The model under review builds one solid part; all positions refer to its coordinate system, in mm. Face numbers are marked on the shaded views. A direction names the side the tool comes from. Coordinates: 2 decimals unless noted, no trailing zeros. Loops run counter-clockwise (first coordinate to the right, second up) from the corner with the lowest first, then second, coordinate; pieces in that order, holes last. Notation, with made-up numbers: (23, 88) - (33, 88) arc R36 ccw to (33, 125) - close; hole circle Ø1 at (38, 28.25). An arc over 180 degrees is marked (long way). One line per item, written item: value. Start each with the question number.
1. We need section C-C, the plane x = -2. Give the boundary of the cut face in (y, z), then the cut area to 3 significant figures.
2. We need section A-A, the plane y = -11.25. Give the boundary of the cut face in (x, z).
3. We need section D-D, the plane z = -5. Give the boundary of the cut face in (x, y).
4. To check wall thickness, follow line 1 (Z direction, x = -2, y = -11.5); line 2 (Z direction, x = 1.5, y = -11); line 3 (Z direction, x = 1.5, y = -0.5). State the ranges of each line that lie inside material, in increasing order.
5. We need section B-B, the plane y = -6. Give the boundary of the cut face in (x, z), then the cut area to 3 significant figures.
6. For the marked faces 5, 6, 7 and 8, list the 3-axis set-ups (+Z, -Z, +X, -X, +Y, -Y) from which the entire face can be reached by the end or side of a thin tool; tool diameter is ignored.
7. Mouldability with a two-part tool opening along Z and no side actions: class the marked faces 1, 2, 3 and 4 as +Z half, -Z half, draft (parallel to the pull), parting line (faces both ways), or undercut.
8. Insertion check: P1, Ø5.5, axis at x = 1.5, z = 15, coming from the -Y side; P2, Ø2, axis at x = 0.78, z = 14.47, coming from the -Y side; P3, Ø1, axis at x = 6, y = -4, coming from the -Z side; P4, Ø2, axis at x = 0.5, z = 3.5, coming from the -Y side. Each pin has a flat end and moves straight along its axis. Give the tip position at first contact, or say it passes through.
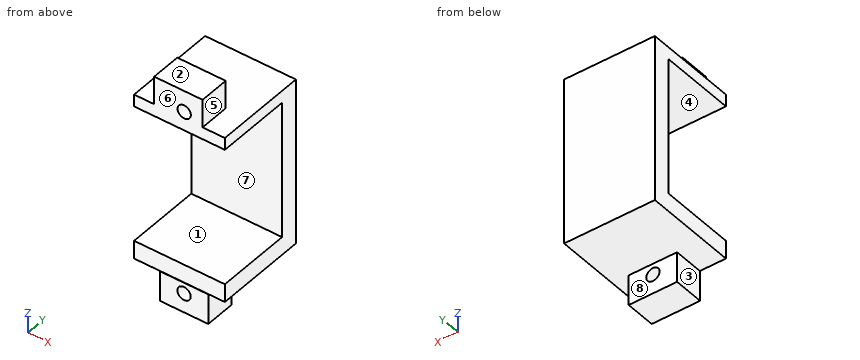
Autodesk Inventor part; units mm, degrees
ref_plane "YZ Plane" through (0, 0, 0) normal (1, 0, 0) x (0, 1, 0)
ref_plane "XZ Plane" through (0, 0, 0) normal (0, 1, 0) x (-1, 0, 0)
ref_plane "XY Plane" through (0, 0, 0) normal (0, 0, 1) x (1, 0, 0)
sketch "Sketch1" plane through (0, 0, 0) normal (0, 1, 0) x (-1, 0, 0)
  line L0 (7.5, 11.35) -> (-7.5, 11.35)
  line L1 (-7.5, 11.35) -> (-7.5, -11.35)
  line L2 (-7.5, -11.35) -> (7.5, -11.35)
  line L3 (7.5, -11.35) -> (7.5, 11.35)
  line L4 (7.5, 11.35) -> (-7.5, -11.35) construction
  line L5 (-7.5, 11.35) -> (7.5, -11.35) construction
  point P0 (0, 0)
  dimension "d0" = 15
  dimension "d1" = 22.7
extrude "Extrusion1" add sketch "Sketch1" along normal blind 3
sketch "Sketch2" plane through (0, 3, 0) normal (0, 1, 0) x (1, 0, 0)
  line L0 (-7.5, 11.35) -> (-7.5, -11.35)
  line L1 (-7.5, -11.35) -> (7.5, -11.35)
  line L2 (7.5, -11.35) -> (7.5, -13.35)
  line L3 (7.5, -13.35) -> (-7.5, -13.35)
  line L4 (-7.5, -13.35) -> (-7.5, -11.35)
  line L5 (-7.5, 11.35) -> (7.5, 11.35)
  line L6 (7.5, 11.35) -> (7.5, 14.35)
  line L7 (7.5, 14.35) -> (-7.5, 14.35)
  line L8 (-7.5, 14.35) -> (-7.5, 11.35)
  point P0 (0, 0)
  dimension "d4" = 15
  dimension "d5" = 2
  dimension "d6" = 3
extrude "Extrusion2" add sketch "Sketch2" against normal blind 15.4
sketch "Sketch3" plane through (-7.5, 3, 13.35) normal (0, 0, 1) x (1, 0, 0)
  line L0 (3.3204, -10.4) -> (11.3204, -10.4)
  line L1 (11.3204, -10.4) -> (11.3204, -15.4)
  line L2 (3.3204, -15.4) -> (3.3204, -10.4)
  line L3 (15, -15.4) -> (0, -15.4)
  line L4 (3.3204, -10.4) -> (7.5, -15.4) construction
  line L5 (11.3204, -10.4) -> (7.5, -15.4) construction
  line L6 (3.3204, -15.4) -> (11.3204, -15.4)
  point P0 (7.5, -3)
  dimension "d9" = 8
  dimension "d10" = 5
extrude "Extrusion3" add sketch "Sketch3" along normal blind 4.65
sketch "Sketch4" plane through (-4.1796, -7.4, 13.35) normal (0, 1, 0) x (1, 0, 0)
  circle A0 centre (4.9615, -1.1239) radius 1.1
  point P0 (4.1796, 13.35)
  dimension "d13" = 2.2
extrude "Extrusion4" cut sketch "Sketch4" against normal blind 6.4
sketch "Sketch5" plane through (7.5, 3, -14.35) normal (0, 0, -1) x (-1, 0, 0)
  line L0 (10.6996, -10.4559) -> (2.6996, -10.4559)
  line L1 (2.6996, -10.4559) -> (2.6996, -15.4559)
  line L2 (10.6996, -15.4559) -> (10.6996, -10.4559)
  line L3 (7.8181, -10.4) -> (7.8181, -15.4)
  line L4 (10.6996, -10.4559) -> (7.8181, -15.4559) construction
  line L5 (2.6996, -10.4559) -> (7.8181, -15.4559) construction
  line L6 (10.6996, -15.4559) -> (2.6996, -15.4559)
  point P0 (7.5, -3)
  point P1 (6.6996, -15.4559)
  point P2 (6.6996, -10.4559)
  dimension "d16" = 8
  dimension "d18" = 5
extrude "Extrusion5" add sketch "Sketch5" along normal blind 5
sketch "Sketch6" plane through (-3.1996, -7.4559, -14.35) normal (0, 1, 0) x (1, 0, 0)
  circle A0 centre (3.9961, 1.8138) radius 1.1
  point P0 (3.1996, -14.35)
  dimension "d21" = 2.2
extrude "Extrusion6" cut sketch "Sketch6" against normal blind 5
properties part number "Sostiene motor_3DPrint"
Findings below:
1. outline: (-12.46, -19.35) - (-7.46, -19.35) - (-7.46, -14.35) - (3, -14.35) - (3, 13.35) - (-7.4, 13.35) - (-7.4, 18) - (-12.4, 18) - (-12.4, 11.35) - (0, 11.35) - (0, -11.35) - (-12.4, -11.35) - (-12.4, -14.35) - (-12.46, -14.35) - close
1. area: 193 mm2
2. outline: (-7.5, -14.35) - (-3.2, -14.35) - (-3.2, -19.35) - (4.8, -19.35) - (4.8, -14.35) - (7.5, -14.35) - (7.5, -11.35) - (-7.5, -11.35) - close; (-7.5, 11.35) - (7.5, 11.35) - (7.5, 13.35) - (3.82, 13.35) - (3.82, 18) - (-4.18, 18) - (-4.18, 13.35) - (-7.5, 13.35) - close; hole circle Ø2.2 at (0.78, 14.47); hole circle Ø2.2 at (0.8, -16.16)
3. outline: (-7.5, 0) - (7.5, 0) - (7.5, 3) - (-7.5, 3) - close
4. line 1: -19.35 to -11.35, 11.35 to 18
4. line 2: -19.35 to -17.01, -15.32 to -11.35, 11.35 to 13.64, 15.31 to 18
4. line 3: -14.35 to -11.35, 11.35 to 13.35
5. outline: (-7.5, -14.35) - (7.5, -14.35) - (7.5, -11.35) - (-7.5, -11.35) - close; (-7.5, 11.35) - (7.5, 11.35) - (7.5, 13.35) - (-7.5, 13.35) - close
5. area: 75.0 mm2
6. face 5: +Z, +X, +Y, -Y
6. face 6: +Z, +X, -X, -Y
6. face 7: +X, -X, -Y
6. face 8: -Z, +X, -X, +Y
7. face 1: undercut
7. face 2: +Z half
7. face 3: draft
7. face 4: undercut
8. P1: y = -12.4
8. P2: through
8. P3: z = -14.35
8. P4: y = 0
